from build123d import *

# Parameters (mm, degrees)
F1_DEPTH = 8
F2_R     = 17.5
F2_R_2   = 5
F3_DEPTH = 8
F4_DEPTH = 8
F6_D     = 5


with BuildPart() as f1:
    # F0 (on Front) → F1 (new body, symmetric)
    with BuildSketch(Plane.XZ):
        with BuildLine():
            Line((17.5, -8), (17.5, 0))
            ThreePointArc((17.5, 0), (0, -17.5), (-17.5, 0))
            Line((-17.5, 0), (-17.5, -8))
            ThreePointArc((-17.5, -8), (-18.671573, -10.828427), (-21.5, -12))
            Line((-21.5, -12), (-31.5, -12))
            ThreePointArc((-31.5, -12), (-32.914214, -12.585786), (-33.5, -14))
            Line((-33.5, -14), (-33.5, -18))
            Line((-33.5, -18), (33.5, -18))
            Line((33.5, -18), (33.5, -14))
            ThreePointArc((33.5, -14), (32.914214, -12.585786), (31.5, -12))
            Line((31.5, -12), (21.5, -12))
            ThreePointArc((21.5, -12), (18.671573, -10.828427), (17.5, -8))
        make_face()
    extrude(amount=F1_DEPTH, both=True)

    # F2 (on Front) → F3 (join)
    with BuildSketch(Plane.XZ):
        Circle(F2_R)
        Circle(F2_R_2, mode=Mode.SUBTRACT)
    extrude(amount=F3_DEPTH)

    # F2 (on Front) → F4 (join)
    with BuildSketch(Plane.XZ):
        Circle(F2_R)
        Circle(F2_R_2, mode=Mode.SUBTRACT)
    extrude(amount=-F4_DEPTH)

    # F6 (through all)
    with Locations(Plane.XY):
        with Locations((-26.5, 0), (26.5, 0)):
            Hole(F6_D / 2)


solid = f1.part
Work out the finished part from the listing and answer in its coordinate system (mm). A direction names the side the tool comes from. Round coordinates to 2 decimals unless told otherwise and drop trailing zeros. Write each loop counter-clockwise with the first axis right and the second up, starting at its lowest first coordinate (ties: lowest second). Pieces come first, ordered by that corner, then holes.
1) A cutting plane is placed at A-A (y = 5.75). Give the vertices of the cut face in (x, z), plus the area to 3 significant figures.
2) A cutting plane is placed at B-B (x = 0). Give the vertices of the cut face in (y, z), plus the area to 3 significant figures.
3) Given pin 1 Ø9 at (y, z) = (-3, -4.5) entering from -X; pin 2 Ø5 at (x, y) = (-28, -3.5) entering from +Z; pin 3 Ø5 at (y, z) = (-4, 13) entering from +X, each flat-ended and moving along its own axis, determine where each tip first touches the part or whether it passes through.
4) The mould has two halves that part along X. Classify faces 4 (the flat face through (0, -8, -8)), 5 (the cylindrical face through (32.93, -0.11, -12.6)), 6 (the flat face through (-33.5, 0, -16)), 7 (the cylindrical face through (29, 0, -15)): pulls with the +X half, pulls with the -X half, needs draft (parallel to the pull), parting line crosses it, or undercut.
5) A cutting plane is placed at C-C (z = 3). Give the vertices of the cut face in (x, y), plus the area to 3 significant figures.
6) A tool of negligible diameter and unlimited length cuts with its end or side. For faces 1 (the cylindrical face through (-24, 0, -15)), 2 (the flat face through (-17.5, 0, -4)), 3 (the flat face through (24, -2, -12)), from which of +Z, -Z, +X, -X, +Y, -Y can it reach the whole face along a straight path? Write none if from no direction.
7) Straight lines are drawn through the part: line 1 (Z direction, x = 0, y = 1.5); line 2 (Y direction, x = 26.5, z = -14.7); line 3 (X direction, y = -6.75, z = 4.5). For each, find the intervals that lie inside material, in ascending order.
8) A cutting plane is placed at D-D (x = -15.5). Give the vertices of the cut face in (y, z).
Completed:
1. outline: (-33.5, -18) - (33.5, -18) - (33.5, -14) arc R2 ccw to (31.5, -12) - (21.5, -12) arc R4 cw to (17.5, -8) - (17.5, 0) arc R17.5 ccw to (-17.5, 0) - (-17.5, -8) arc R4 cw to (-21.5, -12) - (-31.5, -12) arc R2 ccw to (-33.5, -14) - close; hole circle Ø10 at (0, 0)
1. area: 1,230 mm2
2. outline: (-8, -18) - (8, -18) - (8, -5) - (-8, -5) - close; (-8, 5) - (8, 5) - (8, 17.5) - (-8, 17.5) - close
2. area: 408 mm2
3. pin 1: stops at x = -17.63
3. pin 2: stops at z = -12
3. pin 3: stops at x = 14
4. face 4: needs draft
4. face 5: pulls with the +X half
4. face 6: pulls with the -X half
4. face 7: undercut
5. outline: (-17.24, -8) - (-4, -8) - (-4, 8) - (-17.24, 8) - close; (4, -8) - (17.24, -8) - (17.24, 8) - (4, 8) - close
5. area: 424 mm2
6. face 1: +Z, -Z
6. face 2: +Z, -X, +Y, -Y
6. face 3: +Z, +X, +Y, -Y
7. line 1: z = -18 to -5, 5 to 17.5
7. line 2: y = -8 to -2.5, 2.5 to 8
7. line 3: x = -16.91 to -2.18, 2.18 to 16.91
8. outline: (-8, -18) - (8, -18) - (8, 8.12) - (-8, 8.12) - close
